Source: three-view drawing plus pictorial views. Frame: mm from the lowest corner of the part. A direction names the side the tool comes from. Coordinates: 2 decimals unless noted, no trailing zeros. Write each loop counter-clockwise with the first axis right and the second up, starting at its lowest first coordinate (ties: lowest second). Pieces come first, ordered by that corner, then holes. Notation, with made-up numbers: (-2, 50) - (55, 50) arc R16 cw to (55, 79) - close; hole circle Ø8 at (-34.5, 44.25). An arc over 180 degrees is marked (long way). One line per item, written item: value.
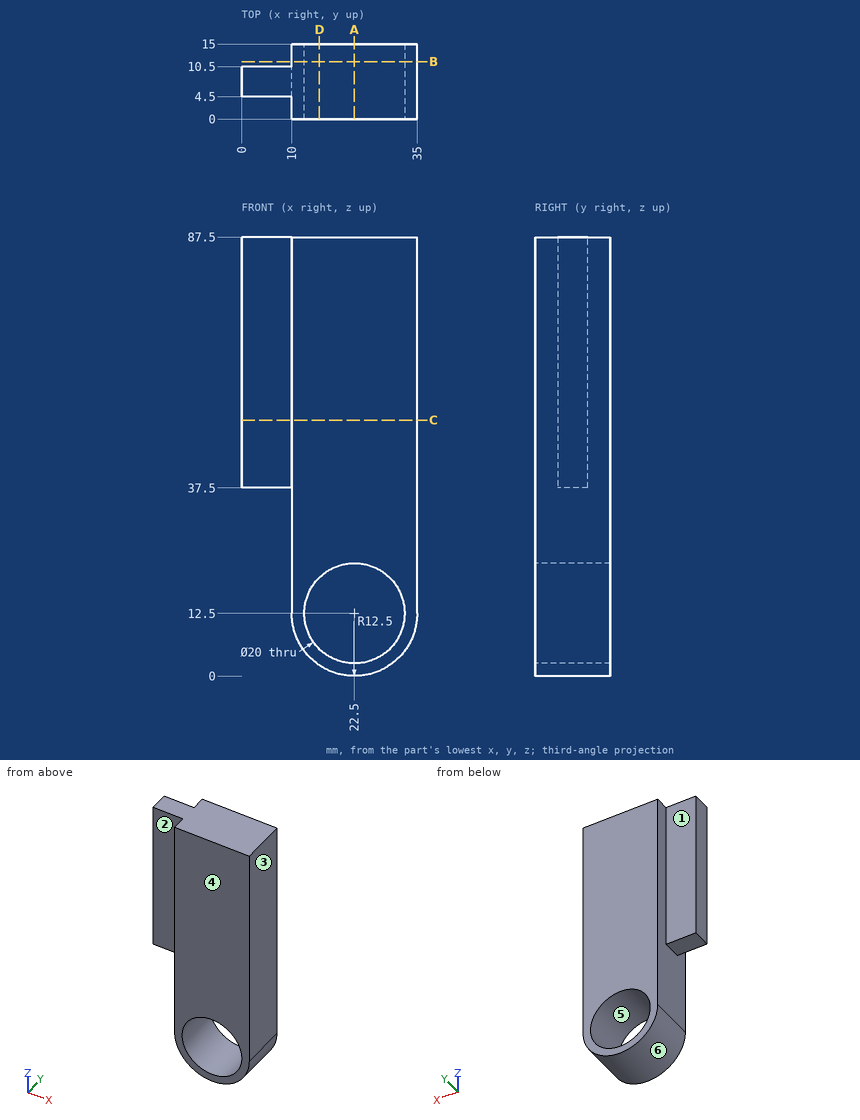
1) Reachability of the marked faces 1, 2 and 3 from +Z, -Z, +X, -X, +Y, -Y: full face, straight path, thin tool, end or side. Return the list, or none.
Values found:
face 1: +Z, -Z, -X, +Y
face 2: +Z, -Z, -X, -Y
face 3: +Z, -Z, +X, +Y, -Y
2) Section query B-B on y = 11.5. Output: boundary loops of the cut face in (x, z), then the cut area to 3 significant figures.
Values found:
outline: (10, 12.5) arc R12.5 ccw to (35, 12.5) - (35, 87.5) - (10, 87.5) - close; hole circle Ø20 at (22.5, 12.5)
area: 1,810 mm2
3) Contact query for flat-ended pins moving along their axis: P1, Ø1.8, axis at x = 6, y = 8.5, coming from the -Z side; P2, Ø3, axis at x = 6.5, z = 51, coming from the -Y side. Output: stop coordinate, or through.
Values found:
P1: z = 37.5
P2: y = 4.5
4) Material intervals for line 1 (Z direction, x = 22.5, y = 5); line 2 (X direction, y = 4.25, z = 70); line 3 (X direction, y = 4, z = 15.5), sorted ascending.
Values found:
line 1: 0 to 2.5, 22.5 to 87.5
line 2: 10 to 35
line 3: 10 to 12.96, 32.04 to 35
5) Section query A-A on x = 22.5. Output: boundary loops of the cut face in (y, z).
Values found:
outline: (0, 0) - (15, 0) - (15, 2.5) - (0, 2.5) - close; (0, 22.5) - (15, 22.5) - (15, 87.5) - (0, 87.5) - close
6) Section query C-C on z = 51. Output: boundary loops of the cut face in (x, y).
Values found:
outline: (0, 4.5) - (10, 4.5) - (10, 0) - (35, 0) - (35, 15) - (10, 15) - (10, 10.5) - (0, 10.5) - close
7) Section query D-D on x = 15.5. Output: boundary loops of the cut face in (y, z), then the cut area to 3 significant figures.
Values found:
outline: (0, 2.14) - (15, 2.14) - (15, 5.36) - (0, 5.36) - close; (0, 19.64) - (15, 19.64) - (15, 87.5) - (0, 87.5) - close
area: 1,070 mm2
8) Draft query along Z for the marked faces 4, 5 and 6. Return one class per face: released by +Z, released by -Z, zero draft, split by the parting line, or undercut.
Values found:
face 4: zero draft
face 5: undercut
face 6: released by -Z
